Geometry check sheet. Reference: the model listing, model coordinates, mm. Face numbers are marked on the shaded views. A direction names the side the tool comes from. Coordinates: 2 decimals unless noted, no trailing zeros. Loops run counter-clockwise (first coordinate to the right, second up) from the corner with the lowest first, then second, coordinate; pieces in that order, holes last. Notation, with made-up numbers: (0, 62) - (46, 62) arc R32 cw to (46, 91) - close; hole circle Ø10 at (-1.75, 73.5). An arc over 180 degrees is marked (long way). Write each question's results on one line, items separated by ' | '. Start each with the question number.
(1) Access from +Z, -Z, +X, -X, +Y, -Y to the whole of each face (thin tool, end or side, straight path). Record for the marked faces 1, 2 and 3.
(2) Mould release check, pull along X, two halves, no side actions. Record for the marked faces 4, 5 and 6: pulls with the +X half, pulls with the -X half, needs draft (parallel to the pull), parting line crosses it, or undercut.
(3) Material ranges on probe 1 along Z at (x, y) = (38, 15.2); probe 2 along Z at (x, y) = (47.5, 15.1); probe 3 along Z at (x, y) = (68, 0.9), recorded low to high.
(4) Sectioned sample at C-C (x = 47.5). Enter the section's corners in (y, z), plus the area to 3 significant figures.
(5) Sectioned sample at D-D (z = 19.8). Enter the section's corners in (x, y).
(6) Sectioned sample at B-B (y = 4.75). Enter the section's corners in (x, z).
(7) Go/stop test with flat-tipped pins: pin 1 Ø3 at (y, z) = (5, 3) entering from +X; pin 2 Ø3.5 at (x, z) = (68, 12) entering from -Y; pin 3 Ø4 at (x, z) = (47.5, 12) entering from -Y; pin 4 Ø6.5 at (y, z) = (6, 16.5) entering from -X. Record where each tip stops, or that it passes through.
(8) Sectioned sample at A-A (z = 12). State how many separate pieces and enclosed holes the cut face has, plus the area to 3 significant figures.
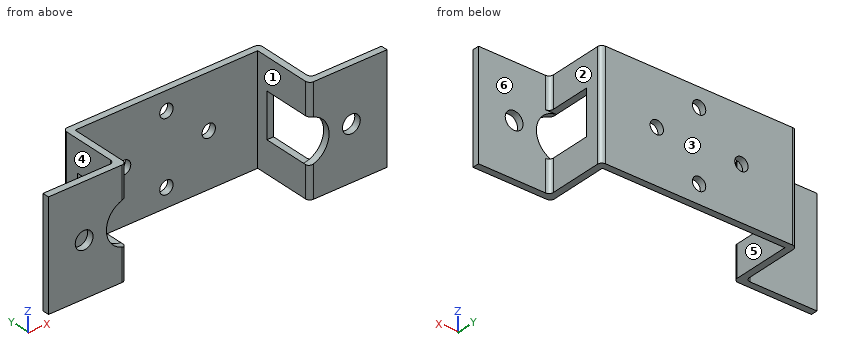
from build123d import *

# Parameters (mm, degrees)
BOSS_EXTRUDE2_DEPTH     = 24
CUT_EXTRUDE1_DEPTH      = 81.91971329657565
CUT_EXTRUDE1_DEPTH_BACK = 81.91971329657565
SKETCH17_R              = 1.9999999999999996
SKETCH17_R_2            = 1.9999999999999962
F_3_0MM_DOWEL_HOLE1_D   = 3
SKETCH22_R              = 5.000000000000001
SKETCH22_R_2            = 4.9999999999999964
CUT_EXTRUDE2_DEPTH      = 1.5
CUT_EXTRUDE3_DEPTH      = 67.45487190567748
CUT_EXTRUDE3_DEPTH_BACK = 67.45487190567748
SKETCH23_W              = 9.949874371066619
SKETCH23_H              = 10
FILLET1_R               = 1


with BuildPart() as part:
    # 3DSketch1 → Boss-Extrude2 (new body)
    with BuildSketch(Plane(origin=(0, 0, 0), x_dir=(0.9998052854172774, 0.01973299905428837, 0), z_dir=(0, -2.14e-15, 1))):
        Polygon((0, 0), (17.496592494802357, -0.34532748345004655), (17.772854481562394, 13.65194651239183), (58.76487118367076, 12.842893551166007), (58.48860919691073, -1.1543804446758696), (75.98520169171307, -1.499707928125916), (76.0148011902945, 2.2e-16), (60.01791662361808, 0.315727984868614), (60.29417861037812, 14.313001980710496), (16.302746052017905, 15.181253939099182), (16.02648406525787, 1.1839799432573024), (0.02959949858143255, 1.4997079281259162), align=None)
    extrude(amount=BOSS_EXTRUDE2_DEPTH)

    # Sketch17 → Cut-Extrude1 (cut, two sides: drawn at the far end of the back side and taken through both)
    with BuildSketch(Plane(origin=(0, 1.5, 0), x_dir=(1, 0, 0), z_dir=(0, 1, 0)).offset(-CUT_EXTRUDE1_DEPTH_BACK)):
        with Locations(Location((8, -12.000000000000002, 0), (0, 0, 270))):
            Circle(SKETCH17_R)
        with Locations(Location((68, -12.000000000000002, 0), (0, 0, 270))):
            Circle(SKETCH17_R_2)
    extrude(amount=CUT_EXTRUDE1_DEPTH + CUT_EXTRUDE1_DEPTH_BACK, mode=Mode.SUBTRACT)

    # Ø3.0mm Dowel Hole1 (through all)
    with Locations(Plane(origin=(-6.1e-16, 15.499999999999996, 0), x_dir=(1, 0, 0), z_dir=(0, 1, 0))):
        with Locations((28.5, -12), (47.5, -12), (38, -19.8), (38, -4.2)):
            Hole(F_3_0MM_DOWEL_HOLE1_D / 2)

    # Sketch22 → Cut-Extrude2 (cut)
    with BuildSketch(Plane(origin=(0, 1.5, 0), x_dir=(1, 0, 0), z_dir=(0, 1, 0))):
        with Locations((17.999999999997943, -12.000000000000927)):
            Circle(SKETCH22_R)
        with Locations((58.00000000000207, -12.000000000000927)):
            Circle(SKETCH22_R_2)
    extrude(amount=-CUT_EXTRUDE2_DEPTH, mode=Mode.SUBTRACT)

    # Sketch23 → Cut-Extrude3 (cut, two sides: drawn at the far end of the back side and taken through both)
    with BuildSketch(Plane.ZY.offset(-16).offset(-CUT_EXTRUDE3_DEPTH_BACK)):
        with Locations((12.000000000000927, 6.5)):
            Rectangle(SKETCH23_W, SKETCH23_H)
    extrude(amount=CUT_EXTRUDE3_DEPTH + CUT_EXTRUDE3_DEPTH_BACK, mode=Mode.SUBTRACT)

    # Fillet1
    fillet1_edges = [part.edges().sort_by_distance(p)[0] for p in [
        (17.500000000000004, -7.53e-15, 3.5125314072338187),
        (17.500000000000004, -4.389e-14, 20.487468592767108),
        (58.50000000000001, -7.53e-15, 3.5125314072338205),
        (58.50000000000001, -4.389e-14, 20.487468592767108),
        (16, 15.499999999999973, 12.000000000000034),
        (60.000000000000014, 15.499999999999975, 12.000000000000034),
        (60.00000000000001, 1.499999999999956, 20.48746859276712),
        (60.00000000000001, 1.4999999999999925, 3.512531407233811),
        (15.999999999999998, 1.4999999999999565, 20.48746859276712),
        (15.999999999999998, 1.499999999999993, 3.5125314072338107),
    ]]
    fillet(fillet1_edges, radius=FILLET1_R)


solid = part.part
Outcome:
1) face 1: +Z, -Z, -Y | face 2: +Z, -Z, +X, +Y | face 3: +Z, -Z, +X, -X, +Y
2) face 4: pulls with the -X half | face 5: undercut | face 6: needs draft
3) probe 1: z = 0 to 2.7, 5.7 to 18.3, 21.3 to 24 | probe 2: z = 0 to 10.5, 13.5 to 24 | probe 3: z = 0 to 10, 14 to 24
4) outline: (14, 0) - (15.5, 0) - (15.5, 10.5) - (14, 10.5) - close; (14, 13.5) - (15.5, 13.5) - (15.5, 24) - (14, 24) - close | area: 31.5 mm2
5) outline: (0, 0) - (16.5, 0) arc R1 ccw to (17.5, 1) - (17.5, 14) - (36.5, 14) - (36.5, 15.5) - (17, 15.5) arc R1 ccw to (16, 14.5) - (16, 2.5) arc R1 cw to (15, 1.5) - (0, 1.5) - close; (39.5, 14) - (58.5, 14) - (58.5, 1) arc R1 ccw to (59.5, 0) - (76, 0) - (76, 1.5) - (61, 1.5) arc R1 cw to (60, 2.5) - (60, 14.5) arc R1 ccw to (59, 15.5) - (39.5, 15.5) - close
6) outline: (16, 0) - (17.5, 0) - (17.5, 7.03) - (16, 7.03) - close; (16, 16.97) - (17.5, 16.97) - (17.5, 24) - (16, 24) - close; (58.5, 0) - (60, 0) - (60, 7.03) - (58.5, 7.03) - close; (58.5, 16.97) - (60, 16.97) - (60, 24) - (58.5, 24) - close
7) pin 1: stops at x = 60 | pin 2: passes through | pin 3: stops at y = 14 | pin 4: stops at x = 16
8) separate pieces: 7 | enclosed holes: 0 | area: 91.1 mm2
